Could you check a few things on this model? Use its own coordinates, in mm. Coordinates: 2 decimals unless noted, no trailing zeros. Loops run counter-clockwise (first coordinate to the right, second up) from the corner with the lowest first, then second, coordinate; pieces in that order, holes last. Notation, with made-up numbers: (-1, 58) - (43, 58) arc R36 cw to (43, 94) - close; hole circle Ø1 at (1.5, 72). An arc over 180 degrees is marked (long way). Use CSV: the item, a comma, the result in double quotes.
from build123d import *

# Parameters (mm, degrees)
SKETCH1_W                    = 88.9
SKETCH1_H                    = 31.75
BASE_FLANGE1_DEPTH           = 6.35
EDGE_FLANGE1_STRIP_CUT_DEPTH = 31.75
EDGE_FLANGE1_DEPTH           = 31.75
TAB1_DEPTH                   = 6.35
SKETCH12_R                   = 4.7625
CUT_EXTRUDE1_DEPTH           = 38.1
SKETCH13_R                   = 4.365625
CUT_EXTRUDE2_DEPTH           = 38.1
BREAK_CORNER1_START          = -6.35
BREAK_CORNER1_DEPTH          = 6.35


# Read off the part's stored shape, not the designer's step: Break-Corner1
# Sheet-metal steps are written as plain solids
with BuildPart() as part:
    # Sketch1 → Base-Flange1 (new body)
    with BuildSketch(Plane.XY):
        Rectangle(SKETCH1_W, SKETCH1_H)
    extrude(amount=-BASE_FLANGE1_DEPTH)

    # Edge-Flange1 strip (across the edge) → Edge-Flange1 strip cut (cut)
    with BuildSketch(Plane(origin=(-44.45, -15.875, -6.35), x_dir=(0.3420201433256631, 0, -0.9396926207859105), z_dir=(0, 1, 0))):
        Polygon((-18.615063745, 32.578309359), (-5.584096284, -3.223979493), (0.382951858, -1.052151583), (-12.648015603, 34.750137269), align=None)
    extrude(amount=EDGE_FLANGE1_STRIP_CUT_DEPTH, mode=Mode.SUBTRACT)

    # Edge-Flange1 section (across the edge) → Edge-Flange1 (add)
    with BuildSketch(Plane(origin=(-44.45, -15.875, -6.35), x_dir=(0.3420201433256631, 0, -0.9396926207859105), z_dir=(0, 1, 0))):
        with BuildLine():
            Line((-6.35, 1.119676327), (-6.35, 94.130323673))
            Line((-6.35, 94.130323673), (0, 94.130323673))
            Line((0, 94.130323673), (0, 1.119676327))
            ThreePointArc((0, 1.119676327), (0.096470768, 0.017010399), (0.382951858, -1.052151583))
            Line((0.382951858, -1.052151583), (-5.584096284, -3.223979493))
            ThreePointArc((-5.584096284, -3.223979493), (-6.157058463, -1.085655529), (-6.35, 1.119676327))
        make_face()
    extrude(amount=EDGE_FLANGE1_DEPTH)

    # Sketch9 → Tab1 (add)
    with BuildSketch(Plane(origin=(-3.158811591, 0, 8.678763518), x_dir=(-0.9396926207859105, 0, -0.342020143325663), z_dir=(0.342020143325663, 0, -0.9396926207859105))):
        Polygon((54.585841232, 15.875), (65.701635901, 31.75), (138.071488577, 31.75), (138.071488577, 15.875), align=None)
        Polygon((138.071488577, -31.75), (138.071488577, -15.875), (54.585841232, -15.875), (65.701635901, -31.75), align=None)
    extrude(amount=-TAB1_DEPTH)

    # Sketch12 → Cut-Extrude1 (cut)
    with BuildSketch(Plane(origin=(-3.158811591, 0, 8.678763518), x_dir=(-0.9396926207859104, 0, -0.34202014332566316), z_dir=(0.34202014332566316, 0, -0.9396926207859104))):
        with Locations((74.424778405, -20.6375)):
            Circle(SKETCH12_R)
        with Locations((125.224778405, -20.6375)):
            Circle(SKETCH12_R)
        with Locations((125.224778405, 20.6375)):
            Circle(SKETCH12_R)
        with Locations((74.424778405, 20.6375)):
            Circle(SKETCH12_R)
    extrude(amount=-CUT_EXTRUDE1_DEPTH, mode=Mode.SUBTRACT)

    # Sketch13 → Cut-Extrude2 (cut)
    with BuildSketch(Plane(origin=(0, 0, -6.35), x_dir=(-1, 0, 0), z_dir=(0, 0, -1))):
        with Locations((28.575, 0)):
            Circle(SKETCH13_R)
        with Locations((-34.925, 0)):
            Circle(SKETCH13_R)
    extrude(amount=-CUT_EXTRUDE2_DEPTH, mode=Mode.SUBTRACT)

    # Break-Corner1 outline → Break-Corner1 (cut)
    with BuildSketch(Plane.XY.offset(BREAK_CORNER1_START)):
        Polygon((44.45, -15.875), (44.45, -9.525), (38.1, -15.875), align=None)
        Polygon((38.1, 15.875), (44.45, 9.525), (44.45, 15.875), align=None)
    extrude(amount=BREAK_CORNER1_DEPTH, mode=Mode.SUBTRACT)


solid = part.part
(1) Please list where these lines run through material, in increasing order: line 1 (Y direction, x = -42, z = -5.5) (3 decimals); line 2 (Z direction, x = -15.5, y = 7).
Computed:
line 1,"y = -15.875 to 15.875"
line 2,"z = -6.35 to 0"
(2) Will these pins go through, and if not, where does the flat tip stop? pin 1 (16 mm diameter, centred on x = 22.5, y = 0.5, fed in from -Z); pin 2 (8 mm diameter, centred on x = 13, z = -4.5, fed in from -Y) (3 decimals); pin 3 (8 mm diameter, centred on x = -54, y = -7.5, fed in from -Z).
Computed:
pin 1,"stops at z = -6.35"
pin 2,"stops at y = -15.875"
pin 3,"stops at z = -11.28"
(3) Suppose I cut it at A-A (y = 0). Write out the boundary of the cut face in (x, z), plus the area to 3 significant figures.
Computed:
outline,"(-135.08, -32.58) - (-132.9, -38.54) - (-45.5, -6.73) arc R6.35 cw to (-43.33, -6.35) - (-32.94, -6.35) - (-32.94, 0) - (-43.33, 0) arc R12.7 ccw to (-47.67, -0.77) - close; (-24.21, -6.35) - (30.56, -6.35) - (30.56, 0) - (-24.21, 0) - close; (39.29, -6.35) - (44.45, -6.35) - (44.45, 0) - (39.29, 0) - close"
area,"1,060 mm²"
(4) Suppose I cut it at D-D (z = -23). Write out the boundary of the cut face in (x, y).
Computed:
outline,"(-108.76, -31.75) - (-90.2, -31.75) - (-90.2, 31.75) - (-108.76, 31.75) - close"
(5) Suppose I cut it at C-C (y = -22.5). Write out the boundary of the cut face in (x, z), plus the area to 3 significant figures.
Computed:
outline,"(-135.08, -32.58) - (-132.9, -38.54) - (-124.95, -35.65) - (-127.12, -29.68) - close; (-118.88, -26.68) - (-116.71, -32.65) - (-77.21, -18.28) - (-79.39, -12.31) - close; (-71.15, -9.31) - (-68.98, -15.28) - (-58.81, -11.58) - (-60.98, -5.61) - close"
area,"389 mm²"
(6) Thinking about a two-plate mould opening in X: for faces 1 (the face through (0, 0, -6.35)), 2 (the face through (-133.974, 0.444, -35.603)), 3 (the face through (-126.04, -22.46, -32.71)), 4 (the face through (41.231, 12.744, -3.219)), which applies, +X half, -X half, draft (parallel to the pull), parting line (faces both ways), or undercut?
Computed:
face 1,"draft"
face 2,"-X half"
face 3,"undercut"
face 4,"+X half"
(7) Suppose I cut it at B-B (x = -121). State how many separate pieces and enclosed holes the cut face has, plus the area to 3 significant figures.
Computed:
separate pieces,"3"
enclosed holes,"0"
area,"304 mm²"
